Autodesk Inventor part; units mm, degrees
ref_plane "Arbeitsebene1" through (-24.9, 0, 0) normal (-1, 0, 0) x (0, 0, 1)
ref_plane "YZ Plane" through (0, 0, 0) normal (1, 0, 0) x (0, 1, 0)
ref_plane "XZ Plane" through (0, 0, 0) normal (0, 1, 0) x (-1, 0, 0)
sketch "Skizze1" plane through (0, 0, 0) normal (0, 1, 0) x (-1, 0, 0)
  line L0 (0, 0) -> (49.8, 0)
  line L1 (49.8, 0) -> (49.8, 9.1)
  line L2 (49.8, 9.1) -> (0, 9.1)
  line L3 (0, 9.1) -> (0, 0)
  line L4 (43.8, 9.1) -> (46.8, 9.1)
  line L5 (46.8, 9.1) -> (46.8, 8.75)
  line L6 (46.8, 8.75) -> (43.8, 8.75)
  line L7 (43.8, 8.75) -> (43.8, 9.1)
  line L8 (59.76, 0) -> (-9.96, 0)
  dimension "d0" = 49.8
  dimension "d1" = 9.1
  dimension "d2" = 3
  dimension "d3" = 3
  dimension "d4" = 0.35
revolve "Umdrehung1" add sketch "Skizze1" angle 360 about axis through (-10, 0, 0) along (1, 0, 0) contours L3 L2 L7 L6 L5 L1 L0
ref_plane "Arbeitsebene1" through (-24.9, 0, 0) normal (-1, 0, 0) x (0, 0, 1)
fillet "Rundung1" radius 2 4 edges at (-46.8, 0, -9.1) (-46.8, 0, -8.75) (-43.8, 0, -8.75) (-43.8, 0, -9.1)
fillet "Rundung2" radius 1 2 edges at (-49.8, 0, -9.1) (0, 0, -9.1)
sketch "Skizze2" plane through (-49.8, 0, 0) normal (-1, 0, 0) x (0, 0, 1)
  circle A0 centre (0, 0) radius 8.1
  circle A1 centre (0, 0) radius 6.5
  dimension "d8" = 13
extrude "Extrusion1" cut sketch "Skizze2" against normal blind 0.2 contours A1
mirror "Spiegeln1" about plane through (-24.9, 0, 0) normal (-1, 0, 0) of "Extrusion1"
sketch "Skizze3" plane through (-49.6, 0, 0) normal (-1, 0, 0) x (0, 0, 1)
  circle A0 centre (0, 0) radius 6.5
  circle A1 centre (0, 0) radius 2.85
  dimension "d11" = 5.7
extrude "Extrusion2" add sketch "Skizze3" along normal blind 1 contours A1
fillet "Rundung3" radius 0.5 1 edges at (-50.6, 0, -2.85)
sketch "Skizze4" plane through (-0.2, 0, 0) normal (1, 0, 0) x (0, 0, -1)
  circle A0 centre (0, 0) radius 6.5
  circle A1 centre (0, 0) radius 5.5
  dimension "d15" = 1
extrude "Extrusion3" add sketch "Skizze4" along normal blind 0.2 contours A1
fillet "Rundung4" radius 0.5 1 edges at (0, 0, 5.5)
properties part number "accu_18500"
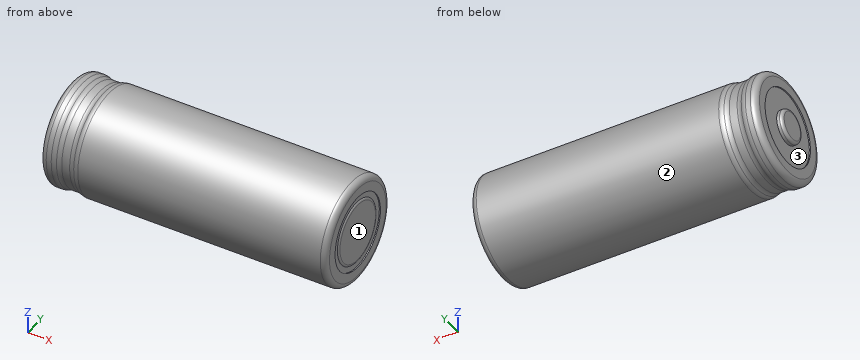
Input: part model. Units: mm. Frame: model coordinates. Face numbers are marked on the shaded views. Give positions to 0.01 mm unless a question says otherwise; leave off trailing zeros. Order: outer loops, then holes, each group sorted by start corner. A loop starts at its lowest first (then second) coordinate and runs counter-clockwise, first axis right, second up.
1. Line query: probe 1 along Y at (x, z) = (-49.7, 0); probe 2 along Y at (x, z) = (-0.1, 0); probe 3 along Y at (x, z) = (-36, -7.25). Output: solid intervals per line, ascending.
Computed:
probe 1: y = -8.54 to -6.5, -2.85 to 2.85, 6.5 to 8.54
probe 2: y = -8.54 to -6.5, -5.4 to 5.4, 6.5 to 8.54
probe 3: y = -5.5 to 5.5
2. Draft query along Z for the marked faces 1, 2 and 3. Return one class per face: released by +Z, released by -Z, zero draft, split by the parting line, or undercut.
Computed:
face 1: zero draft
face 2: split by the parting line
face 3: undercut
3. Cut plane A-A (x = -10.5). Return loops of the section in (y, z), and give its area (3 significant figures).
Computed:
outline: circle Ø18.2 at (0, 0)
area: 260 mm2
4. Pin query (flat end, axial travel): pin 1 Ø2 at (x, y) = (-11, -4.5) entering from -Z; pin 2 Ø2 at (x, y) = (-6.5, 3) entering from -Z; pin 3 Ø1.5 at (x, z) = (-28, 1) entering from -Y. Return the tip coordinate at first contact, or that it passes through.
Computed:
pin 1: stops at z = -8.4
pin 2: stops at z = -8.88
pin 3: stops at y = -9.1
